Autodesk Inventor part; units mm, degrees
ref_plane "YZ Plane" through (0, 0, 0) normal (1, 0, 0) x (0, 1, 0)
ref_plane "XZ Plane" through (0, 0, 0) normal (0, 1, 0) x (-1, 0, 0)
ref_plane "XY Plane" through (0, 0, 0) normal (0, 0, 1) x (1, 0, 0)
sketch "Sketch1" plane through (0, 0, 0) normal (0, 1, 0) x (-1, 0, 0)
  line L0 (0, 0) -> (-19.05, 0)
  line L1 (-19.05, 0) -> (-19.05, -19.05)
  line L2 (-19.05, -19.05) -> (0, -19.05)
  line L3 (0, -19.05) -> (0, 0)
  dimension "d0" = 19.05
  dimension "d1" = 19.05
extrude "Extrusion1" add sketch "Sketch1" along normal blind 101.6
sketch "Sketch2" plane through (19.05, 0, 0) normal (1, 0, 0) x (0, 0, -1)
  line L0 (0, 101.6) -> (19.05, 101.6) construction
  line L1 (9.525, 101.6) -> (9.525, 0) construction
  line L2 (0, 0) -> (19.05, 0) construction
  line L3 (0, 0) -> (0, 101.6) construction
  line L4 (0, 93.0941) -> (19.4916, 93.0941) construction
  circle A0 centre (9.525, 93.0941) radius 3.175
  dimension "d4" = 6.35
extrude "Extrusion2" cut sketch "Sketch2" against normal through all
properties part number "arm holder mount thing"
The listing builds one solid part. Answer for the finished solid, in the listing's coordinates (mm). Give positions to 0.01 mm unless a question says otherwise; leave off trailing zeros. Loops run counter-clockwise (first coordinate to the right, second up) from the corner with the lowest first, then second, coordinate; pieces in that order, holes last. Notation, with made-up numbers: M 51,67.5 L 64,67.5 A18 cw 64,82.5 Z; hole C 44,84 d11. An arc over 180 degrees is marked long. Answer as CSV lines item,"result".
Item 1: The mould has two halves that part along Z. Classify faces 1 (the flat face through (10, 50, -19.05)), 2 (the cylindrical face through (9.658, 90.277, -10.99)), 3 (the flat face through (10, 101.6, -9)): released by +Z, released by -Z, zero draft, split by the parting line, or undercut.
Values follow:
face 1,"released by -Z"
face 2,"undercut"
face 3,"zero draft"
Item 2: The part is cut by section A-A (z = -10). Give the vertices of the cut face in (x, y), and give its area (3 significant figures).
Values follow:
outline,"M 0,0 L 19.05,0 L 19.05,89.95 L 0,89.95 Z; M 0,96.23 L 19.05,96.23 L 19.05,101.6 L 0,101.6 Z"
area,"1,820 mm^2"
Item 3: Straight lines are drawn through the part: line 1 along Z through (x, y) = (14, 95); line 2 along Y through (x, z) = (8.5, -10.5); line 3 along Z through (x, y) = (3.5, 96). For each, find the intervals that lie inside material, in ascending order. Write a range as [from, to].
Values follow:
line 1,"z = [-19.05, -12.06], [-6.99, 0]"
line 2,"y = [0, 90.07], [96.12, 101.6]"
line 3,"z = [-19.05, -10.8], [-8.25, 0]"
Item 4: Given pin 1 Ø5 at (y, z) = (93.09, -9.52) entering from -X, flat-ended and moving along its own axis, determine where the tip first touches the part or whether it passes through.
Values follow:
pin 1,"passes through"
Item 5: The part is cut by section B-B (x = 2). Give the vertices of the cut face in (y, z) (3 decimals).
Values follow:
outline,"M 0,-19.05 L 101.6,-19.05 L 101.6,0 L 0,0 Z; hole C 93.094,-9.525 d6.35"
